For this review, use the dimensioned drawing (mm, ordinates from the lowest corner) and the shaded views. A direction names the side the tool comes from. Coordinates: 2 decimals unless noted, no trailing zeros. Loops run counter-clockwise (first coordinate to the right, second up) from the corner with the lowest first, then second, coordinate; pieces in that order, holes last. Notation, with made-up numbers: (70.5, -28.5) - (108.5, -28.5) arc R17 cw to (108.5, -3.5) - close; hole circle Ø10 at (-29, 33). An arc over 180 degrees is marked (long way). Answer in a Markdown table with one row per item. Add a question column.
(1) Machinability: for the marked faces 1, 2 and 3, which of the approach directions +Z, -Z, +X, -X, +Y, -Y give a long, thin tool a straight path to every point of the face, cutting with its end or side? Answer none if there is none.
(2) We need section A-A on x = 9. Write out the cut boundary in (y, z), plus the area to 3 significant figures.
(3) Mouldability with a two-part tool opening along X and no side actions: class the marked faces 4, 5, 6 and 7 as +X half, -X half, draft (parallel to the pull), parting line (faces both ways), or undercut.
(4) We need section C-C on z = 12. Write out the cut boundary in (x, y), plus the area to 3 significant figures.
(5) We need section D-D on x = 70.5. Write out the cut boundary in (y, z), plus the area to 4 significant figures.
(6) For P1, Ø10, axis at x = 35, z = 6.5, coming from the +Y side; P2, Ø0.6, axis at x = 92, z = 9.5, coming from the +Y side; P3, Ø2.5, axis at y = 55.5, z = 10, coming from the +X side, all flat-tipped, find the tip position at first contact; note any pin that passes through.
(7) We need section B-B on y = 13.5. Write out the cut boundary in (x, z).
(8) For line 1 along X through (y, z) = (37.5, 11); line 2 along Y through (x, z) = (63.5, 14.5); line 3 along Y through (x, z) = (11, 15), list the stretches that pass through material, from the lowest coordinate up.
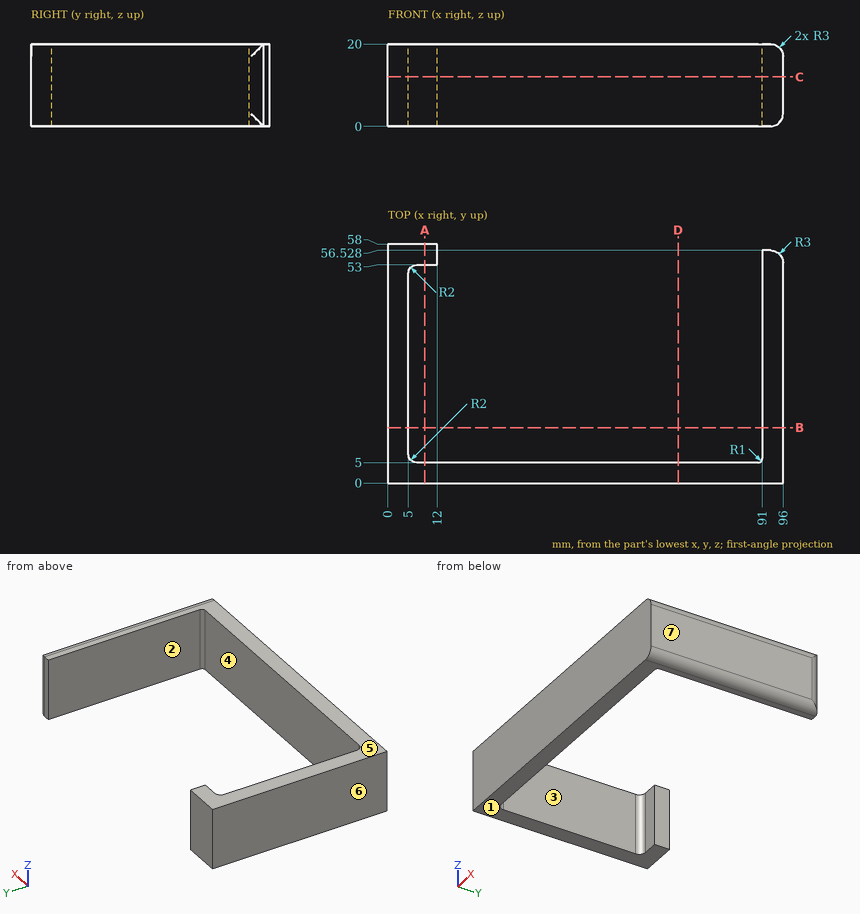
Outcome:
| question | item | result |
|---|---|---|
| 1 | face 1 | -Z, +X, -X, +Y, -Y |
| 1 | face 2 | +Z, -Z, +Y |
| 1 | face 3 | +Z, -Z |
| 2 | outline | (0, 0) - (5, 0) - (5, 20) - (0, 20) - close; (53, 0) - (58, 0) - (58, 20) - (53, 20) - close |
| 2 | area | 200 mm² |
| 3 | face 4 | undercut |
| 3 | face 5 | draft |
| 3 | face 6 | -X half |
| 3 | face 7 | +X half |
| 4 | outline | (0, 0) - (96, 0) - (96, 53.53) arc R3 ccw to (93, 56.53) - (91, 56.53) - (91, 6) arc R1 cw to (90, 5) - (7, 5) arc R2 cw to (5, 7) - (5, 51) arc R2 cw to (7, 53) - (12, 53) - (12, 58) - (0, 58) - close |
| 4 | area | 1,040 mm² |
| 5 | outline | (0, 0) - (5, 0) - (5, 20) - (0, 20) - close |
| 5 | area | 100.0 mm² |
| 6 | P1 | y = 5 |
| 6 | P2 | y = 56.53 |
| 6 | P3 | x = 95.91 |
| 7 | outline | (0, 0) - (5, 0) - (5, 20) - (0, 20) - close; (91, 0) - (93, 0) arc R3 ccw to (96, 3) - (96, 17) arc R3 ccw to (93, 20) - (91, 20) - close |
| 8 | line 1 | 0 to 5, 91 to 96 |
| 8 | line 2 | 0 to 5 |
| 8 | line 3 | 0 to 5, 53 to 58 |
